Could you check a few things on this model? Use its own coordinates, in mm. Face numbers are marked on the shaded views. A direction names the side the tool comes from. Coordinates: 2 decimals unless noted, no trailing zeros. Order: outer loops, then holes, each group sorted by start corner. A loop starts at its lowest first (then second) coordinate and runs counter-clockwise, first axis right, second up. Notation, with made-up numbers: (-30.5, 68.25) - (4.5, 68.25) arc R14 ccw to (4.5, 80.25) - close; hole circle Ø10 at (26, 81). An arc over 180 degrees is marked (long way). One line per item, written item: value.
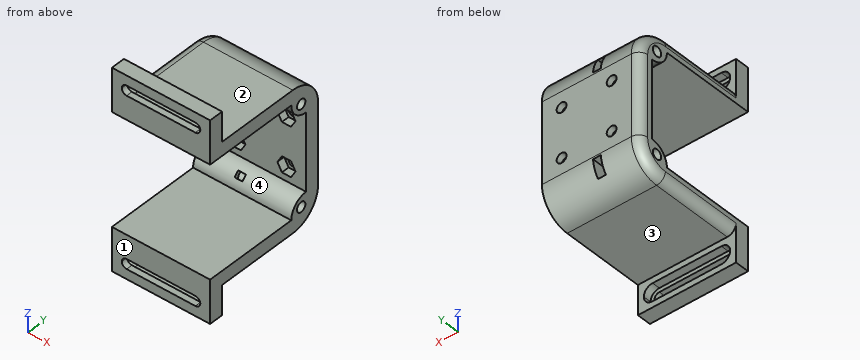
from build123d import *

# Parameters (mm, degrees)
BOSS_EXTRUDE1_DEPTH = 50
SKETCH2_R           = 2.5
CUT_EXTRUDE1_DEPTH  = 50
FILLET1_R           = 15
SKETCH3_W           = 4
SKETCH3_H           = 8
CUT_EXTRUDE2_DEPTH  = 14.54
SKETCH4_W           = 44
SKETCH4_H           = 9
CUT_EXTRUDE3_DEPTH  = 4
SKETCH5_W           = 40
SKETCH5_H           = 5
CUT_EXTRUDE4_DEPTH  = 94.654951818
FILLET2_R           = 2.5
FILLET3_R           = 4.5
FILLET4_R           = 4.5
CUT_EXTRUDE5_START  = -7.129335
SKETCH6_R           = 2.5
CUT_EXTRUDE5_DEPTH  = 4
SKETCH8_R           = 2.5
CUT_EXTRUDE6_DEPTH  = 92.100219539


with BuildPart() as part:
    # Sketch1 → Boss-Extrude1 (new body)
    with BuildSketch(Plane(origin=(0, 0, 0), x_dir=(0, 0, -1), z_dir=(1, 0, 0))):
        with BuildLine():
            Line((35.5, 35.62933491), (-35.5, 35.62933491))
            Line((-35.5, 35.62933491), (-35.5, -21.37066509))
            Line((-35.5, -21.37066509), (-50.5, -21.37066509))
            Line((-50.5, -21.37066509), (-50.5, -28.5))
            Line((-50.5, -28.5), (-28.5, -28.5))
            Line((-28.5, -28.5), (-28.5, 19.7))
            ThreePointArc((-28.5, 19.7), (-22.277460326, 22.277460326), (-19.7, 28.5))
            Line((-19.7, 28.5), (19.7, 28.5))
            ThreePointArc((19.7, 28.5), (22.277460326, 22.277460326), (28.5, 19.7))
            Line((28.5, 19.7), (28.5, -28.5))
            Line((28.5, -28.5), (50.5, -28.5))
            Line((50.5, -28.5), (50.5, -21.37066509))
            Line((50.5, -21.37066509), (35.5, -21.37066509))
            Line((35.5, -21.37066509), (35.5, 35.62933491))
        make_face()
    extrude(amount=BOSS_EXTRUDE1_DEPTH)

    # Sketch2 → Cut-Extrude1 (cut)
    with BuildSketch(Plane.ZY):
        with Locations((-25.5, 25.592902541)):
            Circle(SKETCH2_R)
        with Locations(Location((25.5, 25.592902541, 0), (0, 0, 180))):
            Circle(SKETCH2_R)
    extrude(amount=-CUT_EXTRUDE1_DEPTH, mode=Mode.SUBTRACT)

    # Fillet1
    fillet1_edges = [part.edges().sort_by_distance(p)[0] for p in [
        (25, 35.62933491, 35.5),
        (25, 35.62933491, -35.5),
    ]]
    fillet(fillet1_edges, radius=FILLET1_R)

    # Sketch3 → Cut-Extrude2 (cut)
    with BuildSketch(Plane(origin=(0, 35.62933491, 0), x_dir=(1, 0, 0), z_dir=(0, 1, 0))):
        with Locations((22, 25.5)):
            Rectangle(SKETCH3_W, SKETCH3_H)
        with Locations((22, -25.5)):
            Rectangle(SKETCH3_W, SKETCH3_H)
    extrude(amount=-CUT_EXTRUDE2_DEPTH, mode=Mode.SUBTRACT)

    # Sketch4 → Cut-Extrude3 (cut)
    with BuildSketch(Plane(origin=(0, -21.37066509, 0), x_dir=(1, 0, 0), z_dir=(0, 1, 0))):
        with Locations((25, -43)):
            Rectangle(SKETCH4_W, SKETCH4_H)
        with Locations((25, 43)):
            Rectangle(SKETCH4_W, SKETCH4_H)
    extrude(amount=-CUT_EXTRUDE3_DEPTH, mode=Mode.SUBTRACT)

    # Sketch5 → Cut-Extrude4 (cut, through all)
    with BuildSketch(Plane(origin=(0, -25.37066509, 0), x_dir=(1, 0, 0), z_dir=(0, 1, 0))):
        with Locations((25, -43)):
            Rectangle(SKETCH5_W, SKETCH5_H)
        with Locations((25, 43)):
            Rectangle(SKETCH5_W, SKETCH5_H)
    extrude(amount=-CUT_EXTRUDE4_DEPTH, mode=Mode.SUBTRACT)

    # Fillet2
    fillet2_edges = [part.edges().sort_by_distance(p)[0] for p in [
        (45, -26.935332545, 40.5),
        (45, -26.935332545, 45.5),
        (5, -26.935332545, 45.5),
        (5, -26.935332545, 40.5),
        (5, -26.935332545, -45.5),
        (5, -26.935332545, -40.5),
        (45, -26.935332545, -45.5),
        (45, -26.935332545, -40.5),
    ]]
    fillet(fillet2_edges, radius=FILLET2_R - 0.0001)  # a hair under: the kernel refuses the full size

    # Fillet3
    fillet3_edges = [part.edges().sort_by_distance(p)[0] for p in [
        (3, -23.37066509, 38.5),
        (3, -23.37066509, 47.5),
        (47, -23.37066509, 47.5),
        (47, -23.37066509, 38.5),
        (47, -23.37066509, -47.5),
        (47, -23.37066509, -38.5),
        (3, -23.37066509, -47.5),
        (3, -23.37066509, -38.5),
    ]]
    fillet(fillet3_edges, radius=FILLET3_R - 0.0001)  # a hair under: the kernel refuses the full size

    # Fillet4
    fillet4_edges = [part.edges().sort_by_distance(p)[0] for p in [
        (0, -0.37066509, -35.5),
        (0, -0.37066509, 35.5),
        (0, 35.62933491, 0),
        (0, 31.235936628, -31.106601718),
        (0, 31.235936628, 31.106601718),
    ]]
    fillet(fillet4_edges, radius=FILLET4_R)

    # Sketch6 → Cut-Extrude5 (cut)
    # profile 1 of 4: a face of its own
    with BuildSketch(Plane(origin=(0, 35.62933491, 0), x_dir=(1, 0, 0), z_dir=(0, 1, 0)).offset(CUT_EXTRUDE5_START)):
        Polygon((16.809401077, -8.5), (19.118802154, -12.5), (16.809401077, -16.5), (12.190598923, -16.5), (9.881197846, -12.5), (12.190598923, -8.5), align=None)
        with Locations(Location((14.5, -12.5, 0), (0, 0, 270))):
            Circle(SKETCH6_R, mode=Mode.SUBTRACT)
    # profile 2 of 4: a face of its own
    with BuildSketch(Plane(origin=(0, 35.62933491, 0), x_dir=(1, 0, 0), z_dir=(0, 1, 0)).offset(CUT_EXTRUDE5_START)):
        Polygon((19.118802154, 12.5), (16.809401077, 16.5), (12.190598923, 16.5), (9.881197846, 12.5), (12.190598923, 8.5), (16.809401077, 8.5), align=None)
        with Locations(Location((14.5, 12.5, 0), (0, 0, 270))):
            Circle(SKETCH6_R, mode=Mode.SUBTRACT)
    # profile 3 of 4: a face of its own
    with BuildSketch(Plane(origin=(0, 35.62933491, 0), x_dir=(1, 0, 0), z_dir=(0, 1, 0)).offset(CUT_EXTRUDE5_START)):
        Polygon((42.309401077, -8.5), (37.690598923, -8.5), (35.381197846, -12.5), (37.690598923, -16.5), (42.309401077, -16.5), (44.618802154, -12.5), align=None)
        with Locations(Location((40, -12.5, 0), (0, 0, 270))):
            Circle(SKETCH6_R, mode=Mode.SUBTRACT)
    # profile 4 of 4: a face of its own
    with BuildSketch(Plane(origin=(0, 35.62933491, 0), x_dir=(1, 0, 0), z_dir=(0, 1, 0)).offset(CUT_EXTRUDE5_START)):
        Polygon((37.690598923, 8.5), (35.381197846, 12.5), (37.690598923, 16.5), (42.309401077, 16.5), (44.618802154, 12.5), (42.309401077, 8.5), align=None)
        with Locations(Location((40, 12.5, 0), (0, 0, 270))):
            Circle(SKETCH6_R, mode=Mode.SUBTRACT)
    extrude(amount=CUT_EXTRUDE5_DEPTH, mode=Mode.SUBTRACT)

    # Sketch8 → Cut-Extrude6 (cut, through all)
    with BuildSketch(Plane.XZ.offset(-28.5)):
        with Locations(Location((14.5, -12.5, 0), (0, 0, 270))):
            Circle(SKETCH8_R)
        with Locations(Location((40, 12.5, 0), (0, 0, 270))):
            Circle(SKETCH8_R)
        with Locations(Location((14.5, 12.5, 0), (0, 0, 270))):
            Circle(SKETCH8_R)
        with Locations(Location((40, -12.5, 0), (0, 0, 270))):
            Circle(SKETCH8_R)
    extrude(amount=-CUT_EXTRUDE6_DEPTH, mode=Mode.SUBTRACT)


solid = part.part
Item 1: I want a section at B-B on x = 31. Give the number of separate pieces and of enclosed holes in the cut face, then the cut area to 3 significant figures.
Conclusion:
separate pieces: 3
enclosed holes: 2
area: 1,400 mm²
Item 2: I'm going to push flat-ended pins straight in: pin 1 Ø4.5 at (x, y) = (15, 31.5) entering from -Z; pin 2 Ø6.5 at (x, z) = (14.5, -12.5) entering from -Y; pin 3 Ø6 at (x, y) = (29.5, -12.5) entering from -Z. Where does each tip first touch, or does it pass through?
Conclusion:
pin 1: z = -32.78
pin 2: y = 32.5
pin 3: z = -35.5
Item 3: I want a section at A-A on y = -2. Please give me the cut outline in (x, z), then the cut area to 3 significant figures.
Conclusion:
outline: (0, -31) arc R4.5 ccw to (4.5, -35.5) - (50, -35.5) - (50, -28.5) - (0, -28.5) - close; (0, 28.5) - (50, 28.5) - (50, 35.5) - (4.5, 35.5) arc R4.5 ccw to (0, 31) - close
area: 691 mm²
Item 4: If I drill on probe 1 along X at (y, z) = (26, 29); probe 2 along X at (y, z) = (33.7, 12.5); probe 3 along X at (y, z) = (34.7, 12.5), over which ranges is the centre line in solid material (lowest first)?
Conclusion:
probe 1: 0 to 20, 24 to 50
probe 2: 0.81 to 12, 17 to 37.5, 42.5 to 50
probe 3: 1.76 to 12, 17 to 37.5, 42.5 to 50
Item 5: For the marked faces 1, 2, 3 and 4, which set-ups out of +Z, -Z, +X, -X, +Y, -Y let a thin tool reach every point of the face, with its end or its side?
Conclusion:
face 1: +Z, -Z, +X, -X, -Y
face 2: +Z, +X, -X, +Y
face 3: -Z, +X, -X, +Y
face 4: +X, -X, -Y
Item 6: I want a section at C-C on z = 7. Please give me the cut outline in (x, y).
Conclusion:
outline: (0, 28.5) - (50, 28.5) - (50, 35.63) - (4.5, 35.63) arc R4.5 ccw to (0, 31.13) - close
